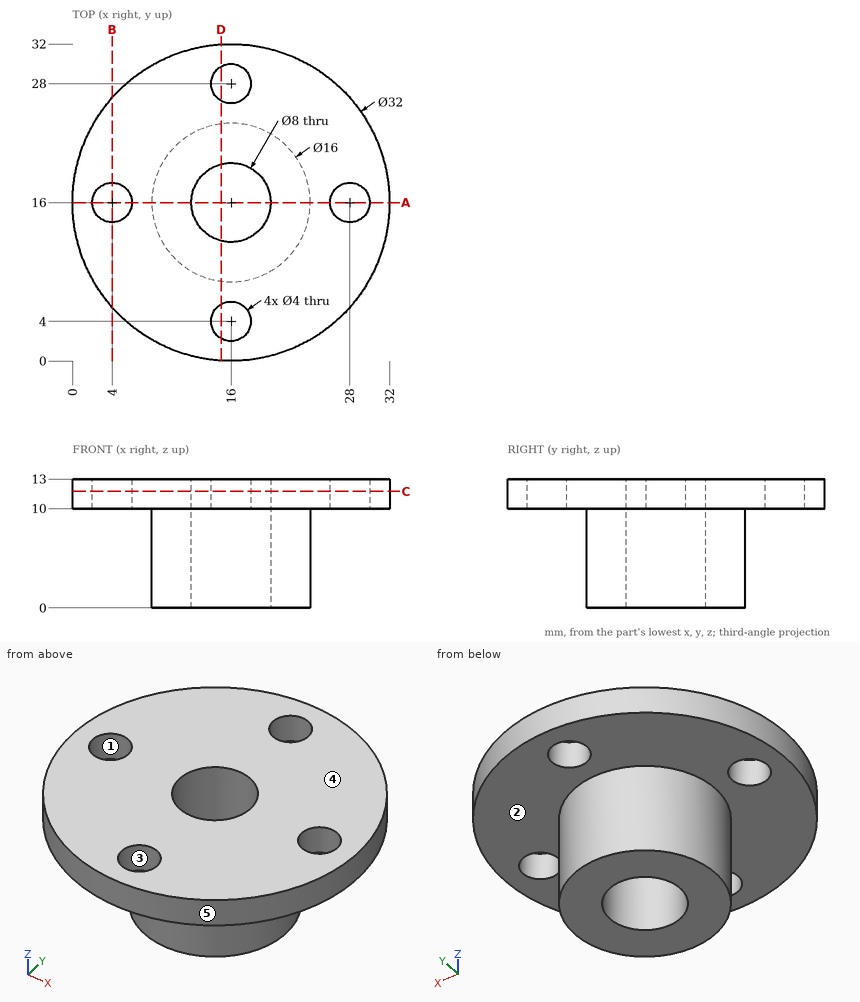
Answer from the drawing. Dimensions are ordinates in mm from the lowest x, y and z of the part. A direction names the side the tool comes from. Give positions to 0.01 mm unless a question says otherwise; leave off trailing zeros. Order: outer loops, then holes, each group sorted by start corner. A loop starts at its lowest first (then second) coordinate and runs counter-clockwise, first axis right, second up. Notation, with made-up numbers: (39, 27) - (86, 27) arc R16 ccw to (86, 56) - close; hole circle Ø7 at (42, 61.25). An arc over 180 degrees is marked (long way). One line per item, written item: value. Start each with the question number.
1) A cutting plane is placed at D-D on x = 15. Give the vertices of the cut face in (y, z).
2) A cutting plane is placed at A-A on y = 16. Give the vertices of the cut face in (x, z), then the cut area to 3 significant figures.
3) The mould has two halves that part along X. Classify the marked faces 3, 4 and 5: released by +X, released by -X, zero draft, split by the parting line, or undercut.
4) Given pin 1 Ø2.5 at (x, y) = (16, 4) entering from -Z; pin 2 Ø5 at (x, y) = (27, 26.5) entering from -Z, each flat-ended and moving along its own axis, determine where each tip first touches the part or whether it passes through.
5) A tool of negligible diameter and unlimited length cuts with its end or side. For the marked faces 1 and 2, from which of +Z, -Z, +X, -X, +Y, -Y can it reach the whole face along a straight path? Write none if from no direction.
6) Find the intervals of material crossed by L1, parallel to X at y = 16, z = 11.45; L2, parallel to X at y = 16, z = 3, in increasing order.
7) A cutting plane is placed at B-B on x = 4. Give the vertices of the cut face in (y, z).
8) A cutting plane is placed at C-C on z = 11.75. Give the vertices of the cut face in (x, y), then the cut area to 3 significant figures.
Answer sheet:
1. outline: (0.03, 10) - (2.27, 10) - (2.27, 13) - (0.03, 13) - close; (5.73, 10) - (8.06, 10) - (8.06, 0) - (12.13, 0) - (12.13, 13) - (5.73, 13) - close; (19.87, 0) - (23.94, 0) - (23.94, 10) - (26.27, 10) - (26.27, 13) - (19.87, 13) - close; (29.73, 10) - (31.97, 10) - (31.97, 13) - (29.73, 13) - close
2. outline: (0, 10) - (2, 10) - (2, 13) - (0, 13) - close; (6, 10) - (8, 10) - (8, 0) - (12, 0) - (12, 13) - (6, 13) - close; (20, 0) - (24, 0) - (24, 10) - (26, 10) - (26, 13) - (20, 13) - close; (30, 10) - (32, 10) - (32, 13) - (30, 13) - close
2. area: 128 mm2
3. face 3: undercut
3. face 4: zero draft
3. face 5: split by the parting line
4. pin 1: passes through
4. pin 2: stops at z = 10
5. face 1: +Z, -Z
5. face 2: -Z
6. L1: x = 0 to 2, 6 to 12, 20 to 26, 30 to 32
6. L2: x = 8 to 12, 20 to 24
7. outline: (5.42, 10) - (14, 10) - (14, 13) - (5.42, 13) - close; (18, 10) - (26.58, 10) - (26.58, 13) - (18, 13) - close
8. outline: circle Ø32 at (16, 16); hole circle Ø4 at (4, 16); hole circle Ø8 at (16, 16); hole circle Ø4 at (16, 4); hole circle Ø4 at (16, 28); hole circle Ø4 at (28, 16)
8. area: 704 mm2
